Input: part model. Units: mm. Frame: model coordinates. A direction names the side the tool comes from. Coordinates: 2 decimals unless noted, no trailing zeros. Order: outer loops, then holes, each group sorted by start corner. A loop starts at its lowest first (then second) coordinate and runs counter-clockwise, first axis right, second up.
from build123d import *

# Parameters (mm, degrees)
SKETCH_1_R               = 9
SKETCH_1_R_2             = 3
EXTRUDE_1_DEPTH          = 15
CUT_EXTRUDE_1_DEPTH      = 5.5
CUT_EXTRUDE_1_DEPTH_BACK = 5.5
SKETCH_3_R               = 18.21
SKETCH_3_R_2             = 8.21


with BuildPart() as part:
    # 草图1 → 凸台-拉伸1 (new body)
    with BuildSketch(Plane.XY):
        Circle(SKETCH_1_R)
        Circle(SKETCH_1_R_2, mode=Mode.SUBTRACT)
    extrude(amount=EXTRUDE_1_DEPTH)

    # 草图3 → 切除-拉伸-薄壁1 (cut, two sides: drawn at the far end of the back side and taken through both)
    with BuildSketch(Plane.XY.offset(7.5).offset(-CUT_EXTRUDE_1_DEPTH_BACK)):
        Circle(SKETCH_3_R)
        Circle(SKETCH_3_R_2, mode=Mode.SUBTRACT)
    extrude(amount=CUT_EXTRUDE_1_DEPTH + CUT_EXTRUDE_1_DEPTH_BACK, mode=Mode.SUBTRACT)


solid = part.part
Item 1: Access query for faces 4 (the face through (3, -8, 2)), 5 (the face through (-1.172, 8.923, 13.986)). Directions: +Z, -Z, +X, -X, +Y, -Y. A direction counts if a zero-diameter tool reaches every point of the face in a straight line with its end or side. Return the directions, or none.
Response values:
face 4: none
face 5: +Z, -Z
Item 2: Pin query (flat end, axial travel): pin 1 Ø1.5 at (x, y) = (1, 0.5) entering from -Z; pin 2 Ø4 at (x, z) = (-6.5, 10) entering from +Y; pin 3 Ø3 at (y, z) = (2, 10.5) entering from -X; pin 4 Ø2 at (x, z) = (0.5, 9) entering from -Y. Return the tip coordinate at first contact, or that it passes through.
Response values:
pin 1: passes through
pin 2: stops at y = 6.87
pin 3: stops at x = -8.19
pin 4: stops at y = -8.21
Item 3: Ray query, probe 1 along Y at (x, z) = (0, 4.25); probe 2 along Y at (x, z) = (2.25, 7.25); probe 3 along X at (y, z) = (-2.5, 7.25). Return the intervals inside material, ascending.
Response values:
probe 1: y = -8.21 to -3, 3 to 8.21
probe 2: y = -7.9 to -1.98, 1.98 to 7.9
probe 3: x = -7.82 to -1.66, 1.66 to 7.82
Item 4: Cut plane C-C on z = 5.25. Return loops of the section in (x, y).
Response values:
outline: circle Ø16.42 at (0, 0); hole circle Ø6 at (0, 0)
Item 5: Cut plane D-D on x = -3.75. Return loops of the section in (y, z).
Response values:
outline: (-8.18, 0) - (8.18, 0) - (8.18, 2) - (7.3, 2) - (7.3, 13) - (8.18, 13) - (8.18, 15) - (-8.18, 15) - (-8.18, 13) - (-7.3, 13) - (-7.3, 2) - (-8.18, 2) - close
Item 6: Draft query along Z for faces 1 (the face through (-3, 0, 7)), 2 (the face through (0, -4, 0)), 3 (the face through (-1.78, -8.015, 7.423)). Return one class per face: pulls with the +Z half, pulls with the -Z half, needs draft (parallel to the pull), parting line crosses it, or undercut.
Response values:
face 1: needs draft
face 2: pulls with the -Z half
face 3: undercut
Item 7: Cut plane A-A on x = 0. Return loops of the section in (y, z), then the cut area to 3 significant figures.
Response values:
outline: (-9, 0) - (-3, 0) - (-3, 15) - (-9, 15) - (-9, 13) - (-8.21, 13) - (-8.21, 2) - (-9, 2) - close; (3, 0) - (9, 0) - (9, 2) - (8.21, 2) - (8.21, 13) - (9, 13) - (9, 15) - (3, 15) - close
area: 163 mm2
